Source: CAD feature listing. Evaluate the final solid. Frame: model axes, mm. A direction names the side the tool comes from. Give positions to 0.01 mm unless a question says otherwise; leave off trailing zeros. Loops run counter-clockwise (first coordinate to the right, second up) from the corner with the lowest first, then second, coordinate; pieces in that order, holes last. Notation, with made-up numbers: M -37.5,83.25 L -27.5,83.25 A14 cw -27.5,105.25 Z; hole C 77.25,80 d1. An arc over 180 degrees is marked long. Put each result on its own line as item: value.
from build123d import *

# Parameters (mm, degrees)
SKETCH2_R               = 3
BOSS_EXTRUDE1_DEPTH     = 180
CUT_EXTRUDE1_DEPTH      = 351.0628515
CUT_EXTRUDE1_DEPTH_BACK = 351.0628515
SKETCH3_W               = 50
SKETCH3_H               = 290
CUT_EXTRUDE2_DEPTH      = 351.0628515
CUT_EXTRUDE2_DEPTH_BACK = 351.0628515
SKETCH4_W               = 102.017694016
SKETCH4_H               = 381.008210697
SKETCH5_W               = 10
SKETCH5_H               = 10
BOSS_EXTRUDE2_DEPTH     = 10
BOSS_EXTRUDE3_REACH     = 309.195
SKETCH6_W               = 10
SKETCH6_H               = 5
SKETCH7_W               = 10
SKETCH7_H               = 10
BOSS_EXTRUDE4_DEPTH     = 30
BOSS_EXTRUDE5_REACH     = 310.95
SKETCH8_W               = 10
SKETCH8_H               = 5
SKETCH9_W               = 30
SKETCH9_H               = 10
BOSS_EXTRUDE6_DEPTH     = 30
FILLET1_R               = 1
CUT_EXTRUDE3_REACH      = 356.718
SKETCH10_R              = 1.5
SKETCH12_R              = 4
BOSS_EXTRUDE7_DEPTH     = 5
SKETCH13_R              = 1.5
CUT_EXTRUDE4_DEPTH      = 355.189214968


with BuildPart() as part:
    # Sketch2 → Boss-Extrude1 (new body)
    with BuildSketch(Plane(origin=(0, 0, 0), x_dir=(0, 0, -1), z_dir=(1, 0, 0))):
        with BuildLine():
            Line((159.16515139, 5), (265.83484861, 5))
            ThreePointArc((265.83484861, 5), (275, 12), (284.16515139, 5))
            Line((284.16515139, 5), (300, 5))
            Line((300, 5), (300, 0))
            Line((300, 0), (284.16515139, 0))
            ThreePointArc((284.16515139, 0), (275, -7), (265.83484861, 0))
            Line((265.83484861, 0), (159.16515139, 0))
            ThreePointArc((159.16515139, 0), (150, -7), (140.83484861, 0))
            Line((140.83484861, 0), (34.16515139, 0))
            ThreePointArc((34.16515139, 0), (25, -7), (15.83484861, 0))
            Line((15.83484861, 0), (0, 0))
            Line((0, 0), (0, 5))
            Line((0, 5), (15.83484861, 5))
            ThreePointArc((15.83484861, 5), (25, 12), (34.16515139, 5))
            Line((34.16515139, 5), (140.83484861, 5))
            ThreePointArc((140.83484861, 5), (150, 12), (159.16515139, 5))
        make_face()
        with Locations(Location((150, 2.5, 0), (0, 0, 180))):
            Circle(SKETCH2_R, mode=Mode.SUBTRACT)
        with Locations(Location((275, 2.5, 0), (0, 0, 180))):
            Circle(SKETCH2_R, mode=Mode.SUBTRACT)
        with Locations(Location((25, 2.5, 0), (0, 0, 180))):
            Circle(SKETCH2_R, mode=Mode.SUBTRACT)
    extrude(amount=BOSS_EXTRUDE1_DEPTH)

    # Sketch3 → Cut-Extrude1 (cut, two sides: drawn at the far end of the back side and taken through both)
    with BuildSketch(Plane(origin=(0, 5, 0), x_dir=(1, 0, 0), z_dir=(0, 1, 0)).offset(-CUT_EXTRUDE1_DEPTH_BACK)):
        with Locations((150, 150)):
            Rectangle(SKETCH3_W, SKETCH3_H)
        with Locations((90, 150)):
            Rectangle(SKETCH3_W, SKETCH3_H)
        with Locations((30, 150)):
            Rectangle(SKETCH3_W, SKETCH3_H)
    extrude(amount=CUT_EXTRUDE1_DEPTH + CUT_EXTRUDE1_DEPTH_BACK, mode=Mode.SUBTRACT)

    # Sketch4 → Cut-Extrude2 (cut, two sides: drawn at the far end of the back side and taken through both)
    with BuildSketch(Plane(origin=(0, 5, 0), x_dir=(1, 0, 0), z_dir=(0, 1, 0)).offset(-CUT_EXTRUDE2_DEPTH_BACK)):
        with Locations((8.991152992, 132.065308574)):
            Rectangle(SKETCH4_W, SKETCH4_H)
    extrude(amount=CUT_EXTRUDE2_DEPTH + CUT_EXTRUDE2_DEPTH_BACK, mode=Mode.SUBTRACT)

    # Sketch5 → Boss-Extrude2 (add)
    with BuildSketch(Plane.XZ):
        with Locations((120, -39.16515139)):
            Rectangle(SKETCH5_W, SKETCH5_H)
        with Locations((180, -39.16515139)):
            Rectangle(SKETCH5_W, SKETCH5_H)
    extrude(amount=BOSS_EXTRUDE2_DEPTH)

    # Sketch6 → Boss-Extrude3 (add, up to next)
    with BuildSketch(Plane(origin=(125, 0, 0), x_dir=(0, 0, -1), z_dir=(1, 0, 0)), mode=Mode.PRIVATE) as boss_extrude3_sk1:
        with Locations((39.16515139, -7.5)):
            Rectangle(SKETCH6_W, SKETCH6_H)
    boss_extrude3_tool1 = extrude(boss_extrude3_sk1.sketch, amount=BOSS_EXTRUDE3_REACH, mode=Mode.PRIVATE) - part.part
    add(boss_extrude3_tool1.solids().sort_by_distance((125, -7.5, -39.165151))[0])

    # Sketch7 → Boss-Extrude4 (add)
    with BuildSketch(Plane(origin=(0, 5, 0), x_dir=(1, 0, 0), z_dir=(0, 1, 0))):
        with Locations((120, 260.83484861)):
            Rectangle(SKETCH7_W, SKETCH7_H)
        with Locations((180, 260.83484861)):
            Rectangle(SKETCH7_W, SKETCH7_H)
    extrude(amount=BOSS_EXTRUDE4_DEPTH)

    # Sketch8 → Boss-Extrude5 (add, up to next)
    with BuildSketch(Plane(origin=(125, 0, 0), x_dir=(0, 0, -1), z_dir=(1, 0, 0)), mode=Mode.PRIVATE) as boss_extrude5_sk1:
        with Locations((260.83484861, 32.5)):
            Rectangle(SKETCH8_W, SKETCH8_H)
    boss_extrude5_tool1 = extrude(boss_extrude5_sk1.sketch, amount=BOSS_EXTRUDE5_REACH, mode=Mode.PRIVATE) - part.part
    add(boss_extrude5_tool1.solids().sort_by_distance((125, 32.5, -260.834849))[0])

    # Sketch9 → Boss-Extrude6 (add)
    with BuildSketch(Plane(origin=(0, -5, 0), x_dir=(1, 0, 0), z_dir=(0, 1, 0))):
        with Locations((149.626726127, 39.16515139)):
            Rectangle(SKETCH9_W, SKETCH9_H)
    extrude(amount=BOSS_EXTRUDE6_DEPTH)

    # Fillet1
    fillet1_edges = [part.edges().sort_by_distance(p)[0] for p in [
        (175, 30, -260.83484861),
        (125, 30, -260.83484861),
    ]]
    fillet(fillet1_edges, radius=FILLET1_R)

    # Sketch10 → Cut-Extrude3 (cut, up to next)
    with BuildSketch(Plane.XZ.offset(-30), mode=Mode.PRIVATE) as cut_extrude3_sk1:
        with Locations(Location((159.960341314, -260.025208151, 0), (0, 0, 270))):
            Circle(SKETCH10_R)
    cut_extrude3_tool1 = extrude(cut_extrude3_sk1.sketch, amount=-CUT_EXTRUDE3_REACH, mode=Mode.PRIVATE) & part.part
    # Sketch10 → Cut-Extrude3 (cut, up to next)
    with BuildSketch(Plane.XZ.offset(-30), mode=Mode.PRIVATE) as cut_extrude3_sk2:
        with Locations(Location((140.127008814, -260.025208151, 0), (0, 0, 270))):
            Circle(SKETCH10_R)
    cut_extrude3_tool2 = extrude(cut_extrude3_sk2.sketch, amount=-CUT_EXTRUDE3_REACH, mode=Mode.PRIVATE) & part.part
    add(cut_extrude3_tool1.solids().sort_by_distance((159.960341, 30, -260.025208))[0], mode=Mode.SUBTRACT)
    add(cut_extrude3_tool2.solids().sort_by_distance((140.127009, 30, -260.025208))[0], mode=Mode.SUBTRACT)

    # Sketch12 → Boss-Extrude7 (add)
    with BuildSketch(Plane(origin=(0, 0, 0), x_dir=(-1, 0, 0), z_dir=(0, -1, 0))):
        with Locations((-62.5, 48)):
            Circle(SKETCH12_R)
        with Locations((-117.5, 48)):
            Circle(SKETCH12_R)
        with BuildLine():
            Line((-85, -1.5), (-95, -1.5))
            ThreePointArc((-95, -1.5), (-99, 2.5), (-95, 6.5))
            Line((-95, 6.5), (-85, 6.5))
            ThreePointArc((-85, 6.5), (-81, 2.5), (-85, -1.5))
        make_face()
    extrude(amount=-BOSS_EXTRUDE7_DEPTH)

    # Sketch13 → Cut-Extrude4 (cut, through all)
    with BuildSketch(Plane(origin=(0, 0, 0), x_dir=(-1, 0, 0), z_dir=(0, -1, 0))):
        with Locations(Location((-62.5, 48, 0), (0, 0, 90))):
            Circle(SKETCH13_R)
        with Locations(Location((-85, 3, 0), (0, 0, 90))):
            Circle(SKETCH13_R)
        with Locations(Location((-95, 3, 0), (0, 0, 90))):
            Circle(SKETCH13_R)
        with Locations(Location((-117.5, 48, 0), (0, 0, 90))):
            Circle(SKETCH13_R)
    extrude(amount=-CUT_EXTRUDE4_DEPTH, mode=Mode.SUBTRACT)


solid = part.part
1. Contact query for flat-ended pins moving along their axis: P1, Ø4, axis at y = 21.5, z = -269, coming from the +X side; P2, Ø1, axis at x = 145.5, y = 24.5, coming from the +Z side; P3, Ø8, axis at y = 2.5, z = -275, coming from the -X side; P4, Ø2.5, axis at x = 181.5, z = -261.5, coming from the -Y side. Output: stop coordinate, or through.
Found:
P1: through
P2: z = -34.17
P3: x = 60
P4: y = 5
2. Access query for faces 5 (the cylindrical face through (58.5, 2.5, -47.9)), 6 (the flat face through (119, 5, -295)), 7 (the flat face through (65, 7, -25)). Directions: +Z, -Z, +X, -X, +Y, -Y. A direction counts if a zero-diameter tool reaches every point of the face in a straight line with its end or side. Return the directions, or none.
Found:
face 5: -X, +Y, -Y
face 6: -Z, +X, -X, +Y
face 7: +Y, -Y
3. Material intervals for line 1 (X direction, y = -2.5, z = -272.5); line 2 (X direction, y = 1.35, z = -3); line 3 (X direction, y = 1, z = -48), sorted ascending. Write a range as from..to.
Found:
line 1: 60..65, 115..125, 175..180
line 2: 60..83.5, 86.5..93.5, 96.5..180
line 3: 58.5..61, 64..66.5, 113.5..116, 119..125, 175..180
4. Draft query along Y for faces 1 (the cylindrical face through (119.9, 2.4, -278)), 2 (the flat face through (120, 0, -213)), 3 (the cylindrical face through (119.9, 2.4, -28)), 4 (the flat face through (63, 5, -88)). Return one class per face: pulls with the +Y half, pulls with the -Y half, needs draft (parallel to the pull), parting line crosses it, or undercut.
Found:
face 1: undercut
face 2: pulls with the -Y half
face 3: undercut
face 4: pulls with the +Y half
5. Section query C-C (z = -106). Output: boundary loops of the cut face in (x, y).
Found:
outline: M 60,0 L 65,0 L 65,5 L 60,5 Z; M 115,0 L 125,0 L 125,5 L 115,5 Z; M 175,0 L 180,0 L 180,5 L 175,5 Z
6. Section query B-B (x = 147.5). Output: boundary loops of the cut face in (y, z), plus the area to 3 significant figures.
Found:
outline: M -10,-44.17 L 25,-44.17 L 25,-34.17 L -10,-34.17 Z; M 0,-300 L 5,-300 L 5,-295 L 0,-295 Z; M 0,-5 L 5,-5 L 5,0 L 0,0 Z; M 30,-265.83 L 35,-265.83 L 35,-255.83 L 30,-255.83 Z
area: 450 mm^2
7. Section query D-D (z = -25). Output: boundary loops of the cut face in (x, y).
Found:
outline: M 60,-7 L 65,-7 L 65,-0.5 L 60,-0.5 Z; M 60,5.5 L 65,5.5 L 65,12 L 60,12 Z; M 115,-7 L 125,-7 L 125,-0.5 L 115,-0.5 Z; M 115,5.5 L 125,5.5 L 125,12 L 115,12 Z; M 175,-7 L 180,-7 L 180,-0.5 L 175,-0.5 Z; M 175,5.5 L 180,5.5 L 180,12 L 175,12 Z
8. Section query A-A (y = 19.5). Output: boundary loops of the cut face in (x, z).
Found:
outline: M 115,-265.83 L 125,-265.83 L 125,-255.83 L 115,-255.83 Z; M 134.63,-44.17 L 164.63,-44.17 L 164.63,-34.17 L 134.63,-34.17 Z; M 175,-265.83 L 185,-265.83 L 185,-255.83 L 175,-255.83 Z
